Geometry check sheet. Reference: the model listing, model coordinates, mm. A direction names the side the tool comes from. Give positions to 0.01 mm unless a question says otherwise; leave off trailing zeros. Write each loop counter-clockwise with the first axis right and the second up, starting at its lowest first coordinate (ties: lowest second). Pieces come first, ordered by that corner, then holes. Notation, with made-up numbers: (-34.75, 74) - (-14.75, 74) arc R36 ccw to (-14.75, 112) - close; hole circle Ø10 at (50, 32.5). An arc over 180 degrees is marked (long way). Use a Markdown table: item, result.
```python
from build123d import *

# Parameters (mm, degrees)
SKETCH_1_W          = 30.8
SKETCH_1_H          = 6.5
EXTRUDE_1_DEPTH     = 8.5
SKETCH_2_R          = 1
CUT_EXTRUDE_1_DEPTH = 2.5
CUT_EXTRUDE_2_REACH = 32.8
SKETCH_3_W          = 7
SKETCH_3_H          = 3.3
FILLET_1_R          = 0.8


with BuildPart() as part:
    # 草图1 → 凸台-拉伸1 (new body, symmetric)
    with BuildSketch(Plane.XY):
        Rectangle(SKETCH_1_W, SKETCH_1_H)
    extrude(amount=EXTRUDE_1_DEPTH, both=True)

    # 草图2 → 切除-拉伸1 (cut)
    with BuildSketch(Plane(origin=(0, 3.25, 0), x_dir=(1, 0, 0), z_dir=(0, 1, 0))):
        with Locations((-6.5, 6)):
            Circle(SKETCH_2_R)
        with Locations((-6.5, -6)):
            Circle(SKETCH_2_R)
        with Locations((6.5, 6)):
            Circle(SKETCH_2_R)
        with Locations((6.5, -6)):
            Circle(SKETCH_2_R)
    extrude(amount=-CUT_EXTRUDE_1_DEPTH, mode=Mode.SUBTRACT)

    # 草图3 → 切除-拉伸2 (cut, up to next)
    with BuildSketch(Plane.ZY.offset(15.4), mode=Mode.PRIVATE) as cut_extrude_2_sk1:
        with Locations((0, -1.6)):
            Rectangle(SKETCH_3_W, SKETCH_3_H)
    cut_extrude_2_tool1 = extrude(cut_extrude_2_sk1.sketch, amount=-CUT_EXTRUDE_2_REACH, mode=Mode.PRIVATE) & part.part
    add(cut_extrude_2_tool1.solids().sort_by_distance((-15.4, -1.6, 0))[0], mode=Mode.SUBTRACT)

    # 圆角1
    fillet_1_edges = [part.edges().sort_by_distance(p)[0] for p in [
        (0, 3.25, 8.5),
        (15.4, -3.25, -6),
        (-15.4, -3.25, -6),
        (0, 3.25, -8.5),
        (0, -3.25, -8.5),
        (0, -3.25, 8.5),
        (-15.4, 3.25, 0),
        (15.4, 3.25, 0),
        (15.4, -3.25, 6),
        (-15.4, -3.25, 6),
    ]]
    fillet(fillet_1_edges, radius=FILLET_1_R)


solid = part.part
```
1) Depth check by flat-ended pin: P1, Ø0.6, axis at x = -6.5, z = 6, coming from the +Y side; P2, Ø3.5, axis at x = 4.5, z = 0, coming from the -Y side. Enter the tip coordinate at first touch or a pass-through.
Working result:
| item | result |
|---|---|
| P1 | stops at y = 0.75 |
| P2 | stops at y = 0.05 |
2) Section check C-C on y = 1.75. Record the boundary of the cut face in (x, z).
Working result:
| item | result |
|---|---|
| outline | (-15.4, -8.5) - (15.4, -8.5) - (15.4, 8.5) - (-15.4, 8.5) - close; hole circle Ø2 at (-6.5, -6); hole circle Ø2 at (-6.5, 6); hole circle Ø2 at (6.5, -6); hole circle Ø2 at (6.5, 6) |
3) Section check A-A on y = -0.25. Record the boundary of the cut face in (x, z), then the cut area to 3 significant figures.
Working result:
| item | result |
|---|---|
| outline | (-15.4, -8.5) - (15.4, -8.5) - (15.4, -3.5) - (-15.4, -3.5) - close; (-15.4, 3.5) - (15.4, 3.5) - (15.4, 8.5) - (-15.4, 8.5) - close |
| area | 308 mm² |
4) Mould release check, pull along X, two halves, no side actions. Record for faces 1 (the flat face through (0, -3.25, 6)), 2 (the cylindrical face through (15.16, -3.02, 6.04)), 3 (the flat face through (-7, 0.75, 6)): pulls with the +X half, pulls with the -X half, needs draft (parallel to the pull), parting line crosses it, or undercut.
Working result:
| item | result |
|---|---|
| face 1 | needs draft |
| face 2 | pulls with the +X half |
| face 3 | undercut |
5) Section check B-B on x = -6.5. Record the boundary of the cut face in (y, z), then the cut area to 3 significant figures.
Working result:
| item | result |
|---|---|
| outline | (-3.25, -7.7) arc R0.8 ccw to (-2.45, -8.5) - (2.45, -8.5) arc R0.8 ccw to (3.25, -7.7) - (3.25, -7) - (0.75, -7) - (0.75, -5) - (3.25, -5) - (3.25, 5) - (0.75, 5) - (0.75, 7) - (3.25, 7) - (3.25, 7.7) arc R0.8 ccw to (2.45, 8.5) - (-2.45, 8.5) arc R0.8 ccw to (-3.25, 7.7) - (-3.25, 3.5) - (0.05, 3.5) - (0.05, -3.5) - (-3.25, -3.5) - close |
| area | 76.9 mm² |
6) Section check D-D on z = -0.5. Record the boundary of the cut face in (x, y).
Working result:
| item | result |
|---|---|
| outline | (-15.4, 0.05) - (15.4, 0.05) - (15.4, 2.45) arc R0.8 ccw to (14.6, 3.25) - (-14.6, 3.25) arc R0.8 ccw to (-15.4, 2.45) - close |
7) Set-up check for faces 4 (the flat face through (0, 0.05, 0)), 5 (the cylindrical face through (-7.237, 2.018, 5.324)), 6 (the cylindrical face through (15.16, 3.02, -0.12)): record each of +Z, -Z, +X, -X, +Y, -Y from which the full face is reachable in a straight line by a thin tool's end or side.
Working result:
| item | result |
|---|---|
| face 4 | +X, -X, -Y |
| face 5 | +Y |
| face 6 | +Z, -Z, +X, +Y |
8) Material ranges on L1, parallel to Z at x = -6.5, y = 2.05; L2, parallel to X at y = 2.45, z = -6; L3, parallel to Z at x = -5.5, y = -0.5, recorded low to high. Write a range as from..to.
Working result:
| item | result |
|---|---|
| L1 | z = -8.5..-7, -5..5, 7..8.5 |
| L2 | x = -15.4..-7.5, -5.5..5.5, 7.5..15.4 |
| L3 | z = -8.5..-3.5, 3.5..8.5 |
